```python
from build123d import *

# Parameters (mm, degrees)
F0_R     = 4
F1_DEPTH = 5


with BuildPart() as f1:
    # F0 (on Top) → F1 (new body)
    with BuildSketch(Plane.XY):
        with BuildLine():
            ThreePointArc((2.499999978, -4.3301270316), (4.3301270126, -2.500000011), (5, 0))
            ThreePointArc((5, 0), (4.330127022, 2.4999999946), (2.5000000107, 4.3301270127))
            ThreePointArc((2.5000000107, 4.3301270127), (-3.05e-08, 5), (-2.5000000636, 4.3301269822))
            ThreePointArc((-2.5000000636, 4.3301269822), (-4.3301270373, 2.4999999682), (-5, 0))
            ThreePointArc((-5, 0), (-4.3301270351, -2.4999999721), (-2.5000000559, -4.3301269867))
            ThreePointArc((-2.5000000559, -4.3301269867), (-4.5e-08, -5), (2.499999978, -4.3301270316))
        make_face()
        Circle(F0_R, mode=Mode.SUBTRACT)
        with BuildLine():
            Line((5, -2.8867513459), (5, 0))
            ThreePointArc((5, 0), (4.3301270126, -2.500000011), (2.499999978, -4.3301270316))
            Line((2.499999978, -4.3301270316), (5, -2.8867513459))
        make_face()
        with BuildLine():
            ThreePointArc((2.5000000107, 4.3301270127), (4.330127022, 2.4999999946), (5, 0))
            Line((5, 0), (5, 2.8867513459))
            Line((5, 2.8867513459), (2.5000000107, 4.3301270127))
        make_face()
        with BuildLine():
            ThreePointArc((-2.5000000636, 4.3301269822), (-3.05e-08, 5), (2.5000000107, 4.3301270127))
            Line((2.5000000107, 4.3301270127), (0, 5.7735026919))
            Line((0, 5.7735026919), (-2.5000000636, 4.3301269822))
        make_face()
        with BuildLine():
            Line((0, -5.7735026919), (2.499999978, -4.3301270316))
            ThreePointArc((2.499999978, -4.3301270316), (-4.5e-08, -5), (-2.5000000559, -4.3301269867))
            Line((-2.5000000559, -4.3301269867), (0, -5.7735026919))
        make_face()
        with BuildLine():
            ThreePointArc((-5, 0), (-4.3301270373, 2.4999999682), (-2.5000000636, 4.3301269822))
            Line((-2.5000000636, 4.3301269822), (-5, 2.8867513459))
            Line((-5, 2.8867513459), (-5, 0))
        make_face()
        with BuildLine():
            Line((-5, -2.8867513459), (-2.5000000559, -4.3301269867))
            ThreePointArc((-2.5000000559, -4.3301269867), (-4.3301270351, -2.4999999721), (-5, 0))
            Line((-5, 0), (-5, -2.8867513459))
        make_face()
    extrude(amount=F1_DEPTH)


solid = f1.part
```
Geometry check sheet. Reference: the model listing, model coordinates, mm. Round coordinates to 2 decimals unless told otherwise and drop trailing zeros. Write each loop counter-clockwise with the first axis right and the second up, starting at its lowest first coordinate (ties: lowest second). Pieces come first, ordered by that corner, then holes. Notation, with made-up numbers: (-3.5, 73.25) -> (37.5, 73.25) arc R24 cw to (37.5, 85.25) -> close; hole circle Ø6 at (11.5, 39.5). An arc over 180 degrees is marked (long way). Put each result on its own line as item: value.
1) Cross-section at A-A, the plane y = 0. Enter the section's corners in (x, z), plus the area to 3 significant figures.
Recorded:
outline: (-5, 0) -> (-4, 0) -> (-4, 5) -> (-5, 5) -> close; (4, 0) -> (5, 0) -> (5, 5) -> (4, 5) -> close
area: 10.0 mm2
2) Cross-section at B-B, the plane z = 2.6. Enter the section's corners in (x, y).
Recorded:
outline: (-5, -2.89) -> (0, -5.77) -> (5, -2.89) -> (5, 2.89) -> (0, 5.77) -> (-5, 2.89) -> close; hole circle Ø8 at (0, 0)
3) Depth check by flat-ended pin: P1, Ø1, axis at x = -2, z = 2.5, coming from the -Y side. Enter the tip coordinate at first touch or a pass-through.
Recorded:
P1: stops at y = -4.91
4) Release check for a two-part mould opening along X. For faces 1 (the face through (5, 0, 2)), 2 (the face through (-0.867, -3.905, 2.465)), 3 (the face through (-3, -3, 5)) record: pulls with the +X half, pulls with the -X half, needs draft (parallel to the pull), parting line crosses it, or undercut.
Recorded:
face 1: pulls with the +X half
face 2: undercut
face 3: needs draft
5) Cross-section at D-D, the plane y = 4.5. Enter the section's corners in (x, z), plus the area to 3 significant figures.
Recorded:
outline: (-2.21, 0) -> (2.21, 0) -> (2.21, 5) -> (-2.21, 5) -> close
area: 22.1 mm2
6) Cross-section at C-C, the plane x = -0.75. Enter the section's corners in (y, z), plus the area to 3 significant figures.
Recorded:
outline: (-5.34, 0) -> (-3.93, 0) -> (-3.93, 5) -> (-5.34, 5) -> close; (3.93, 0) -> (5.34, 0) -> (5.34, 5) -> (3.93, 5) -> close
area: 14.1 mm2
7) Thickness scan on probe 1 along Y at (x, z) = (-0.25, 2.65); probe 2 along Y at (x, z) = (-3.5, 0.55); probe 3 along X at (y, z) = (3, 0.45). Record the ranges inside material, lowest first. Write a range as from..to.
Recorded:
probe 1: y = -5.63..-3.99, 3.99..5.63
probe 2: y = -3.75..-1.94, 1.94..3.75
probe 3: x = -4.8..-2.65, 2.65..4.8
